```python
from build123d import *

# Parameters (mm, degrees)
SKETCH011_R  = 1.5
PAD004_DEPTH = 10
PAD002_DEPTH = 3


with BuildPart() as armmountcutout:
    # Sketch011 → Pad004 (new body, symmetric)
    with BuildSketch(Plane.XZ):
        with Locations((-2.25, 21.222956)):
            Circle(SKETCH011_R)
        with Locations((-3.75, 16.222956)):
            Circle(SKETCH011_R)
        with Locations((2.25, 21.222956)):
            Circle(SKETCH011_R)
        with Locations((3.75, 16.222956)):
            Circle(SKETCH011_R)
    extrude(amount=PAD004_DEPTH, both=True)


with BuildPart() as cut002:
    # Sketch009 → Pad002 (new body)
    with BuildSketch(Plane.XZ):
        with BuildLine():
            ThreePointArc((7.761952, 10.442802), (0, 13.011534), (-7.761952, 10.442802))
            Line((-17.297442, 15.597632), (-7.761952, 10.442802))
            Line((-12.220397, 100.442802), (-17.297442, 15.597632))
            ThreePointArc((-12.220397, 100.442802), (0, 89.783571), (12.220397, 100.442802))
            Line((17.297442, 15.597632), (12.220397, 100.442802))
            Line((7.761952, 10.442802), (17.297442, 15.597632))
        make_face()
    extrude(amount=-PAD002_DEPTH)

    # Cut002: cut ArmMountCutout
    add(armmountcutout.part, mode=Mode.SUBTRACT)


solid = cut002.part
```
Source: CAD feature listing. Evaluate the final solid. Frame: model axes, mm. Coordinates: 2 decimals unless noted, no trailing zeros. Loops run counter-clockwise (first coordinate to the right, second up) from the corner with the lowest first, then second, coordinate; pieces in that order, holes last. Notation, with made-up numbers: M 71.5,15 L 121.5,15 A22 ccw 121.5,37 Z; hole C 17,21.25 d5. An arc over 180 degrees is marked long. Use CSV: the item, a comma, the result in double quotes.
(1) Contact query for flat-ended pins moving along their axis: pin 1 (2.5 mm diameter, centred on x = 3.75, z = 16.22, fed in from -Y); pin 2 (1 mm diameter, centred on y = 2, z = 44, fed in from -X); pin 3 (1 mm diameter, centred on y = 1.5, z = 21, fed in from -X). Output: stop coordinate, or through.
Answers follow:
pin 1,"through"
pin 2,"x = -15.63"
pin 3,"x = -17"
(2) Line query: line 1 (X direction, y = 0.4, z = 16); line 2 (Z direction, x = -5, y = 2.3); line 3 (Z direction, x = -5.5, y = 1.35). Output: solid intervals per line, ascending. Write a range as [from, to].
Answers follow:
line 1,"[-17.27, -5.23], [-2.27, 2.27], [5.23, 17.27]"
line 2,"[12.01, 15.39], [17.05, 90.84]"
line 3,"[11.79, 91.08]"
(3) Cut plane A-A on y = 1.55. Return loops of the section in (x, z), and give its area (3 significant figures).
Answers follow:
outline,"M -17.3,15.6 L -7.76,10.44 A13.01 cw 7.76,10.44 L 17.3,15.6 L 12.22,100.44 A12.33 cw -12.22,100.44 Z; hole C -3.75,16.22 d3; hole C -2.25,21.22 d3; hole C 2.25,21.22 d3; hole C 3.75,16.22 d3"
area,"2,380 mm²"
(4) Cut plane B-B on z = 67. Return loops of the section in (x, y).
Answers follow:
outline,"M -14.22,0 L 14.22,0 L 14.22,3 L -14.22,3 Z"
(5) Draft query along X for faces 1 (the face through (0.12, 1.48, 13.01)), 2 (the face through (12.463, 1.479, 12.984)), 3 (the face through (-12.6, 1.48, 13.06)), 4 (the face through (5.136, 1.479, 15.648)). Return one class per face: pulls with the +X half, pulls with the -X half, needs draft (parallel to the pull), parting line crosses it, or undercut.
Answers follow:
face 1,"undercut"
face 2,"pulls with the +X half"
face 3,"pulls with the -X half"
face 4,"undercut"
(6) Cut plane C-C on x = 13. Return loops of the section in (y, z).
Answers follow:
outline,"M 0,13.27 L 3,13.27 L 3,87.41 L 0,87.41 Z"
